from build123d import *

# Parameters (mm, degrees)
SCHIZZO1_W                   = 5
SCHIZZO1_H                   = 2.8
ESTRUSIONE_ESTRUSIONE1_DEPTH = 7
ESTRUSIONE_ESTRUSIONE2_DEPTH = 2
RACCORDO1_R                  = 2
SCHIZZO3_W                   = 0.7
SCHIZZO3_H                   = 0.7
ESTRUSIONE_ESTRUSIONE3_DEPTH = 0.5
SCHIZZO4_W                   = 1.74
SCHIZZO4_H                   = 0.7
SCHIZZO4_W_2                 = 0.7
ESTRUSIONE_ESTRUSIONE4_DEPTH = 0.8
SCHIZZO5_W                   = 0.7
SCHIZZO5_H                   = 0.7
ESTRUSIONE_ESTRUSIONE5_DEPTH = 1.9
SCHIZZO6_R                   = 0.35
ESTRUSIONE_ESTRUSIONE6_DEPTH = 3


with BuildPart() as part:
    # Schizzo1 → Estrusione-Estrusione1 (new body)
    with BuildSketch(Plane(origin=(0, 0, 0), x_dir=(1, 0, 0), z_dir=(0, 1, 0))):
        with Locations((2.5, 1.4)):
            Rectangle(SCHIZZO1_W, SCHIZZO1_H)
    extrude(amount=ESTRUSIONE_ESTRUSIONE1_DEPTH)

    # Schizzo2 → Estrusione-Estrusione2 (add)
    with BuildSketch(Plane.XY):
        with BuildLine():
            Line((0.5, 0), (4.5, 0))
            Line((4.5, 0), (4.5, 4.5))
            ThreePointArc((4.5, 4.5), (2.5, 6.5), (0.5, 4.5))
            Line((0.5, 4.5), (0.5, 0))
        make_face()
    extrude(amount=ESTRUSIONE_ESTRUSIONE2_DEPTH)

    # Raccordo1
    raccordo1_edges = [part.edges().sort_by_distance(p)[0] for p in [
        (4.5, 2.25, 2),
        (0.5, 2.25, 2),
        (2.5, 6.5, 2),
    ]]
    fillet(raccordo1_edges, radius=RACCORDO1_R - 0.0001)  # a hair under: the kernel refuses the full size

    # Schizzo3 → Estrusione-Estrusione3 (add)
    with BuildSketch(Plane(origin=(0, 0, 0), x_dir=(-1, 0, 0), z_dir=(0, -1, 0))):
        with Locations((-1.35, 1.4)):
            Rectangle(SCHIZZO3_W, SCHIZZO3_H)
        with Locations((-2.5, 1.4)):
            Rectangle(SCHIZZO3_W, SCHIZZO3_H)
        with Locations((-3.65, 1.4)):
            Rectangle(SCHIZZO3_W, SCHIZZO3_H)
    extrude(amount=ESTRUSIONE_ESTRUSIONE3_DEPTH)

    # Schizzo4 → Estrusione-Estrusione4 (add)
    with BuildSketch(Plane(origin=(0, -0.5, 0), x_dir=(-1, 0, 0), z_dir=(0, -1, 0))):
        with Locations((-0.83, 1.4)):
            Rectangle(SCHIZZO4_W, SCHIZZO4_H)
        with Locations((-2.5, 1.4)):
            Rectangle(SCHIZZO4_W_2, SCHIZZO4_H)
        with Locations((-4.17, 1.4)):
            Rectangle(SCHIZZO4_W, SCHIZZO4_H)
    extrude(amount=ESTRUSIONE_ESTRUSIONE4_DEPTH)

    # Schizzo5 → Estrusione-Estrusione5 (add)
    with BuildSketch(Plane.XZ.offset(1.3)):
        with Locations((0.31, -1.4)):
            Rectangle(SCHIZZO5_W, SCHIZZO5_H)
        with Locations((4.69, -1.4)):
            Rectangle(SCHIZZO5_W, SCHIZZO5_H)
        with Locations((2.5, -1.4)):
            Rectangle(SCHIZZO5_W, SCHIZZO5_H)
    extrude(amount=ESTRUSIONE_ESTRUSIONE5_DEPTH)

    # Schizzo6 → Estrusione-Estrusione6 (add)
    with BuildSketch(Plane.XZ.offset(3.2)):
        with Locations(Location((0.31, -1.4, 0), (0, 0, 270))):
            Circle(SCHIZZO6_R)
        with Locations(Location((2.5, -1.4, 0), (0, 0, 270))):
            Circle(SCHIZZO6_R)
        with Locations(Location((4.69, -1.4, 0), (0, 0, 270))):
            Circle(SCHIZZO6_R)
    extrude(amount=ESTRUSIONE_ESTRUSIONE6_DEPTH)


solid = part.part
Design review of the part built by this model. Coordinates are the model's own, in mm. A direction names the side the tool comes from. Round coordinates to 2 decimals unless told otherwise and drop trailing zeros. Loops run counter-clockwise (first coordinate to the right, second up) from the corner with the lowest first, then second, coordinate; pieces in that order, holes last. Notation, with made-up numbers: (84.5, 12.5) -> (131.5, 12.5) arc R16 ccw to (131.5, 30.5) -> close; hole circle Ø5 at (1.25, 88.5). An arc over 180 degrees is marked (long way). Use one line per item in the form item = value. Start each with the question number.
Q1. We need section B-B on z = -0.45. Give the boundary of the cut face in (x, y), then the cut area to 3 significant figures.
Q2. Machinability: for faces 1 (the face through (0, 3, -1)), 2 (the face through (1, -1, -1.75)), 3 (the face through (5, 3, -1)), 4 (the face through (1, -1, -1.05)), which of the approach directions +Z, -Z, +X, -X, +Y, -Y give a long, thin tool a straight path to every point of the face, cutting with its end or side? Answer none if there is none.
Q3. We need section A-A on y = -3. Give the boundary of the cut face in (x, z), then the cut area to 3 significant figures.
Q4. For pin 1 Ø3 at (x, y) = (1, -4) entering from -Z; pin 2 Ø1.4 at (y, z) = (2.5, -1) entering from -X; pin 3 Ø1 at (y, z) = (3, 1) entering from +X, all flat-tipped, find the tip position at first contact; note any pin that passes through.
Q5. Wall thickness on line 1 along X through (y, z) = (-1.5, -1.45); line 2 along X through (y, z) = (5.5, -1.8); line 3 along Y through (x, z) = (1.35, -0.25): over which ranges is each line inside the solid? List them lowest first. Write a range as [from, to].
Q6. Draft analysis for pull direction Z (two halves, no side actions). For faces 5 (the face through (2, 7, -1)), 6 (the face through (4, -1, -1.05)), 7 (the face through (4, -1, -1.75)), state which applies: +Z half, -Z half, draft (parallel to the pull), parting line (faces both ways), or undercut.
Calculated:
q1.outline = (0, 0) -> (5, 0) -> (5, 7) -> (0, 7) -> close
q1.area = 35.0 mm²
q2.face_1 = +Z, -Z, -X, +Y
q2.face_2 = -Z, +X, -X, -Y
q2.face_3 = +Z, -Z, +X, +Y
q2.face_4 = +Z, +X, -X, -Y
q3.outline = (-0.04, -1.75) -> (0.66, -1.75) -> (0.66, -1.05) -> (-0.04, -1.05) -> close; (2.15, -1.75) -> (2.85, -1.75) -> (2.85, -1.05) -> (2.15, -1.05) -> close; (4.34, -1.75) -> (5.04, -1.75) -> (5.04, -1.05) -> (4.34, -1.05) -> close
q3.area = 1.47 mm²
q4.pin_1 = -1.75
q4.pin_2 = 0
q4.pin_3 = 4.44
q5.line_1 = [-0.04, 0.66], [2.15, 2.85], [4.34, 5.04]
q5.line_2 = [0, 5]
q5.line_3 = [0, 7]
q6.face_5 = draft
q6.face_6 = +Z half
q6.face_7 = -Z half
